Autodesk Inventor part; units mm, degrees
ref_plane "YZ Plane" through (0, 0, 0) normal (1, 0, 0) x (0, 1, 0)
ref_plane "XZ Plane" through (0, 0, 0) normal (0, 1, 0) x (-1, 0, 0)
ref_plane "XY Plane" through (0, 0, 0) normal (0, 0, 1) x (1, 0, 0)
sketch "Sketch1" plane through (0, 0, 0) normal (0, 0, 1) x (1, 0, 0)
  line L0 (24.605, -18.795) -> (-24.605, -18.795)
  line L1 (-24.605, -18.795) -> (-24.605, 18.795)
  line L2 (-24.605, 18.795) -> (24.605, 18.795)
  line L3 (24.605, 18.795) -> (24.605, -18.795)
  line L4 (26.195, 20.385) -> (-26.195, 20.385)
  line L5 (-26.195, 20.385) -> (-26.195, 18.795)
  line L6 (-26.195, -20.385) -> (-24.605, -20.385)
  line L7 (26.195, -20.385) -> (26.195, 20.385)
  line L8 (24.605, -18.795) -> (24.605, -20.385)
  arc A0 (-26.195, -18.795) -> (-24.605, -20.385) centre (-24.605, -18.795) ccw
  line L9 (-24.605, -20.385) -> (24.605, -20.385)
  line L10 (-26.195, -18.795) -> (-26.195, -20.385)
  line L11 (-24.605, 18.795) -> (-26.195, 18.795)
  line L12 (-26.195, 18.795) -> (-26.195, -18.795)
  line L13 (24.605, -20.385) -> (26.195, -20.385)
  point P0 (0, 0)
  point P1 (0, -18.795)
  point P2 (-24.605, 0)
  dimension "d0" = 49.21
  dimension "d1" = 37.59
  dimension "d2" = 1.59
extrude "Extrusion1" add sketch "Sketch1" against normal blind 37.59 contours L8 L9 A0 L12 L11 L1 L0
sketch "Sketch3" plane through (-24.605, -20.385, 0) normal (0, -1, 0) x (1, 0, 0)
  line L0 (0, -37.59) -> (49.21, -37.59)
  line L1 (49.21, 0) -> (49.21, -37.59)
  line L2 (0, 0) -> (49.21, 0)
  line L3 (0, 0) -> (0, -37.59)
  circle A0 centre (4.76, -3.175) radius 1.59
  circle A1 centre (11.11, -3.175) radius 1.59
  circle A2 centre (17.46, -3.175) radius 1.59
  circle A3 centre (23.81, -3.175) radius 1.59
  circle A4 centre (30.16, -3.175) radius 1.59
  circle A5 centre (36.51, -3.175) radius 1.59
  circle A6 centre (42.86, -3.175) radius 1.59
  arc A7 (49.21, -3.175) -> (46.035, 0) centre (46.035, -3.175) ccw
  line L4 (49.21, -18.795) -> (59.21, -18.795)
  circle A8 centre (4.76, -34.415) radius 1.59
  circle A9 centre (11.11, -34.415) radius 1.59
  circle A10 centre (17.46, -34.415) radius 1.59
  circle A11 centre (23.81, -34.415) radius 1.59
  circle A12 centre (30.16, -34.415) radius 1.59
  circle A13 centre (36.51, -34.415) radius 1.59
  circle A14 centre (42.86, -34.415) radius 1.59
  arc A15 (46.035, -37.59) -> (49.21, -34.415) centre (46.035, -34.415) ccw
  line L5 (46.035, -37.59) -> (49.21, -37.59)
  line L6 (49.21, -34.415) -> (49.21, -37.59)
  line L7 (49.21, -3.175) -> (49.21, 0)
  line L8 (46.035, 0) -> (49.21, 0)
  line L9 (-1.59, 0) -> (-1.59, -37.59)
  line L10 (-1.59, -37.59) -> (0, -37.59)
  line L11 (0, 0) -> (0, -37.59)
  line L12 (-1.59, 0) -> (0, 0)
  line L13 (-1.59, 0) -> (-1.59, -37.59)
  point P0 (24.605, 0)
  dimension "d12" = 6.35
  dimension "d13" = 6.35
  dimension "d14" = 6.35
  dimension "d15" = 6.35
  dimension "d16" = 6.35
  dimension "d17" = 6.35
  dimension "d18" = 6.35
  dimension "d19" = 3.18
  dimension "d20" = 15.62
  dimension "d21" = 10
extrude "Extrusion2" cut sketch "Sketch3" against normal through all contours L3 L2 A7 L1 A15 L0 | L10 L9 L12 L3 keep common part
sketch "Sketch4" plane through (-26.195, -18.795, -37.59) normal (-1, 0, 0) x (0, 0, 1)
  line L0 (0, 37.59) -> (0, 0)
  line L1 (37.59, 0) -> (0, 0)
  line L2 (37.59, 37.59) -> (37.59, 0)
  line L3 (37.59, 37.59) -> (0, 37.59)
  line L4 (1.585, -1.59) -> (4.765, -1.59)
  line L5 (32.825, -1.59) -> (36.005, -1.59)
  line L6 (12.19, 11.785) -> (25.4, 11.785)
  line L7 (25.4, 11.785) -> (25.4, 25.805)
  line L8 (25.4, 25.805) -> (12.19, 25.805)
  line L9 (12.19, 25.805) -> (12.19, 11.785)
  arc A0 (25.4, 25.805) -> (12.19, 25.805) centre (18.795, 25.805) ccw
  arc A1 (12.19, 11.785) -> (25.4, 11.785) centre (18.795, 11.785) ccw
  arc A2 (18.795, 37.59) -> (0, 18.795) centre (18.795, 18.795) ccw
  line L10 (0, 18.795) -> (0, 37.59)
  line L11 (37.59, 37.59) -> (37.59, 18.795)
  line L12 (0, 37.59) -> (37.59, 37.59)
  circle A3 centre (18.795, 18.795) radius 15.5
  circle A4 centre (11.045, 32.2184) radius 1.625
  circle A5 centre (3.295, 18.795) radius 1.625
  circle A6 centre (11.045, 5.3716) radius 1.625
  circle A7 centre (26.545, 5.3716) radius 1.625
  circle A8 centre (34.295, 18.795) radius 1.625
  circle A9 centre (26.545, 32.2184) radius 1.625
  arc A10 (37.59, 18.795) -> (18.795, 37.59) centre (18.795, 18.795) ccw
  arc A11 (0, 18.795) -> (37.59, 18.795) centre (18.795, 18.795) ccw
  point P0 (3.295, 18.795)
  point P1 (26.545, 32.2184)
  point P2 (11.045, 5.3716)
  point P3 (34.295, 18.795)
  point P4 (26.545, 5.3716)
  dimension "d24" = 13.21
  dimension "d25" = 14.02
  dimension "d26" = 12.19
  dimension "d27" = 11.785
  dimension "d28" = 15.5
  dimension "d29" = 15.5
  dimension "d30" = 15.5
  dimension "d31" = 15.5
  dimension "d32" = 15.5
  dimension "d33" = 15.5
  dimension "d34" = 3.25
  dimension "d37" = 360
extrude "Extrusion3" cut sketch "Sketch4" against normal through all contours L3 A2 L0 | L3 L2 A10 | L9 L8 L7 L6 | L6 A1 | A0 L8 | A3 A8 | A3 A8 | A9 A3 | A3 A9 | A7 A3 | A3 A7 | A4 A3 | A3 A4 | A6 A3 | A3 A6 | A5 A3 | A3 A5
equation "\"d13\" = d12"
equation "\"d14\" = d13"
equation "\"d15\" = d14"
equation "\"d16\" = d15"
equation "\"d17\" = d16"
equation "\"d18\" = d17"
properties part number "beslag"
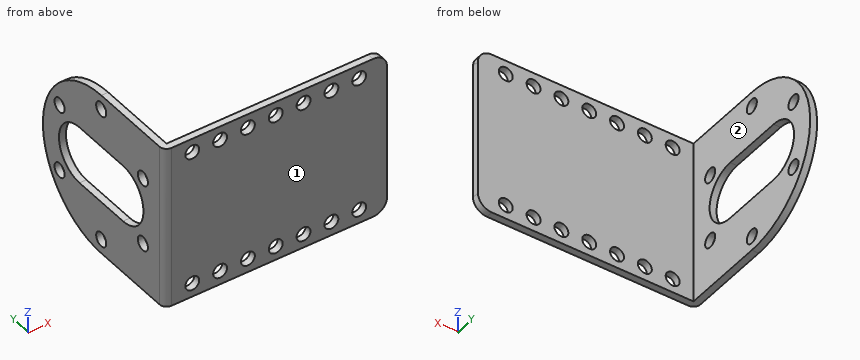
Verification items for the finished model (mm, model axes). Face numbers are marked on the shaded views. A direction names the side the tool comes from. Give positions to 0.01 mm unless a question says otherwise; leave off trailing zeros. Order: outer loops, then holes, each group sorted by start corner. A loop starts at its lowest first (then second) coordinate and runs counter-clockwise, first axis right, second up. Notation, with made-up numbers: M 70.5,72 L 102.5,72 A22 cw 102.5,98 Z; hole C 46.5,24.5 d1. An arc over 180 degrees is marked long. Use one line per item in the form item = value. Start each with the question number.
Q1. Scan lines: line 1 along Y through (x, z) = (-20, -11) (3 decimals); line 2 along X through (y, z) = (-16.5, -23) (3 decimals). Record each from-to range of solid material in increasing order. Write a range as [from, to].
Q2. Access from +Z, -Z, +X, -X, +Y, -Y to the whole of each face (thin tool, end or side, straight path). Record for the marked faces 1 and 2.
Q3. Section check A-A (x = -7). Enter the section's corners in (y, z) (3 decimals), then the cut area to 3 significant figures.
Q4. Section check C-C (y = 11). Enter the section's corners in (x, z) (3 decimals), then the cut area to 3 significant figures.
Q5. Section check B-B (z = -18). Enter the section's corners in (x, y) (3 decimals), then the cut area to 3 significant figures.
Q6. Section check D-D (z = -11.5). Enter the section's corners in (x, y) (3 decimals), then the cut area to 3 significant figures.
Q7. Go/stop test with flat-tipped pins: pin 1 Ø19 at (y, z) = (6.5, -10.5) entering from +X (3 decimals); pin 2 Ø3 at (x, z) = (10.5, -24.5) entering from +Y (3 decimals); pin 3 Ø1.7 at (x, y) = (-25.5, 2) entering from +Z. Record where each tip stops, or that it passes through.
Evaluation:
q1.line_1 = [-20.385, -18.795]
q1.line_2 = [-26.195, -24.605]
q2.face_1 = +Z, -Z, +X, -X, -Y
q2.face_2 = +Z, -Z, +X, +Y
q3.outline = M -20.385,-37.59 L -18.795,-37.59 L -18.795,-35.998 L -20.385,-35.998 Z; M -20.385,-32.832 L -18.795,-32.832 L -18.795,-4.758 L -20.385,-4.758 Z; M -20.385,-1.592 L -18.795,-1.592 L -18.795,0 L -20.385,0 Z
q3.area = 49.7 mm2
q4.outline = M -26.195,-34.035 L -24.605,-34.035 L -24.605,-24.059 L -26.195,-24.059 Z; M -26.195,-13.531 L -24.605,-13.531 L -24.605,-3.555 L -26.195,-3.555 Z
q4.area = 31.7 mm2
q5.outline = M -26.195,-18.795 A1.59 ccw -24.605,-20.385 L 24.605,-20.385 L 24.605,-18.795 L -24.605,-18.795 L -24.605,-13.567 L -26.195,-13.567 Z; M -26.195,13.567 L -24.605,13.567 L -24.605,18.778 L -26.195,18.778 Z
q5.area = 96.8 mm2
q6.outline = M -26.195,-18.795 A1.59 ccw -24.605,-20.385 L 24.605,-20.385 L 24.605,-18.795 L -24.605,-18.795 L -24.605,-14.983 L -26.195,-14.983 Z; M -26.195,-11.863 L -24.605,-11.863 L -24.605,11.863 L -26.195,11.863 Z; M -26.195,14.983 L -24.605,14.983 L -24.605,17.322 L -26.195,17.322 Z
q6.area = 128 mm2
q7.pin_1 = -24.605
q7.pin_2 = -18.795
q7.pin_3 = -0.04
